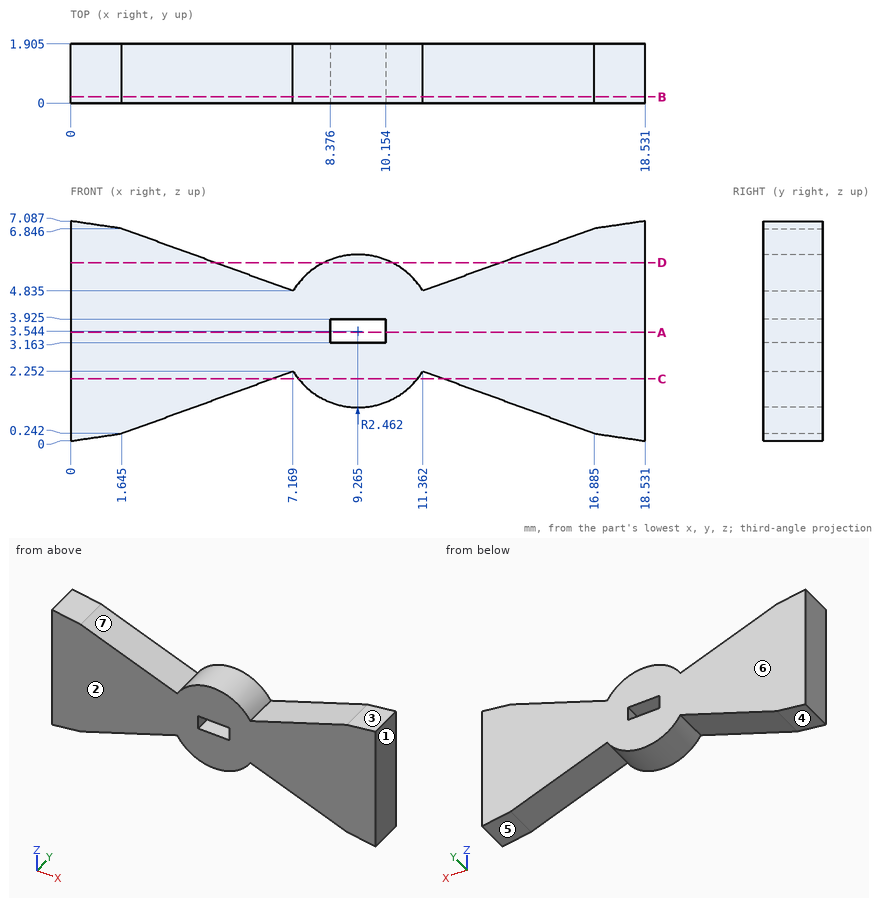
Study the drawing (mm; zero at the part's minimum x, y, z) and answer. A direction names the side the tool comes from. Give positions to 0.01 mm unless a question says otherwise; leave off trailing zeros. Write each loop counter-clockwise with the first axis right and the second up, starting at its lowest first coordinate (ties: lowest second). Pieces come first, ordered by that corner, then holes. Notation, with made-up numbers: M -19,52.25 L 18,52.25 A26 ccw 18,74.25 Z; hole C 76,-18 d10. An arc over 180 degrees is marked long. Put each result on its own line as item: value. Start each with the question number.
1. Consider line 1 along Z through (x, y) = (16.75, 0.4) (1 decimal); line 2 along Z through (x, y) = (7.25, 1.5); line 3 along Z through (x, y) = (9.5, 0.55) (1 decimal). Determine where each line is inside the solid, lowest interval first.
2. The part is cut by section A-A, the plane z = 3.5. Give the vertices of the cut face in (x, y) (1 decimal).
3. The part is cut by section D-D, the plane z = 5.75. Give the vertices of the cut face in (x, y) (1 decimal), and give its area (3 significant figures).
4. The part is cut by section C-C, the plane z = 2. Give the vertices of the cut face in (x, y) (1 decimal).
5. The part is cut by section B-B, the plane y = 0.2. Give the vertices of the cut face in (x, z) (1 decimal).
6. Each of these flat-tipped pins is pushed along its axis until it touches: pin 1 Ø0.9 at (x, y) = (9.5, 1.5) entering from +Z; pin 2 Ø0.9 at (x, y) = (9, 1) entering from -Z; pin 3 Ø1 at (x, y) = (12.5, 1.5) entering from -Z (1 decimal). Where does it stop, or does it pass through?
7. For a pull along X with two mould halves and no side action, classify the marked faces 1, 2, 3 and 4 as released by +X, released by -X, zero draft, split by the parting line, or undercut.
8. Which of the six approach directions +Z, -Z, +X, -X, +Y, -Y give full straight-line access (tool end or side, diameter ignored) to the marked faces 5, 6 and 7?
Final values:
1. line 1: z = 0.3 to 6.8
1. line 2: z = 2.13 to 4.96
1. line 3: z = 1.1 to 3.2, 3.9 to 6
2. outline: M 0,0 L 8.4,0 L 8.4,1.9 L 0,1.9 Z; M 10.2,0 L 18.5,0 L 18.5,1.9 L 10.2,1.9 Z
3. outline: M 0,0 L 4.7,0 L 4.7,1.9 L 0,1.9 Z; M 8.2,0 L 10.4,0 L 10.4,1.9 L 8.2,1.9 Z; M 13.9,0 L 18.5,0 L 18.5,1.9 L 13.9,1.9 Z
3. area: 21.9 mm²
4. outline: M 0,0 L 6.5,0 L 6.5,1.9 L 0,1.9 Z; M 7.3,0 L 11.2,0 L 11.2,1.9 L 7.3,1.9 Z; M 12.1,0 L 18.5,0 L 18.5,1.9 L 12.1,1.9 Z
5. outline: M 0,0 L 1.6,0.2 L 7.2,2.3 A2.5 ccw 11.4,2.3 L 16.9,0.2 L 18.5,0 L 18.5,7.1 L 16.9,6.8 L 11.4,4.8 A2.5 ccw 7.2,4.8 L 1.6,6.8 L 0,7.1 Z; hole M 8.4,3.2 L 10.2,3.2 L 10.2,3.9 L 8.4,3.9 Z
6. pin 1: stops at z = 6.01
6. pin 2: stops at z = 1.08
6. pin 3: stops at z = 1.7
7. face 1: released by +X
7. face 2: zero draft
7. face 3: undercut
7. face 4: undercut
8. face 5: -Z, +Y, -Y
8. face 6: +Z, -Z, +X, -X, +Y
8. face 7: +Z, +Y, -Y
